Build history of the part. All positions in model axes, mm. Face numbers are marked on the shaded views. Coordinates: 2 decimals unless noted, no trailing zeros. One line per item, written item: value. Start each with the question number.
```python
from build123d import *

# Parameters (mm, degrees)
F0_W     = 135.89
F0_H     = 135.89
F1_DEPTH = 31.75


# Not quite as in the source:
# - a fillet or chamfer that OpenCascade refuses, or shapes differently, is made with other operations: its cross-section is extruded or revolved along the edge and cut away or added


with BuildPart() as f1:
    # F0 (on Top) → F1 (new body)
    with BuildSketch(Plane.XY):
        Rectangle(F0_W, F0_H)
    extrude(amount=F1_DEPTH)

    # F2 (on Front) → F3 (revolve, cut)
    with BuildSketch(Plane.XZ):
        with BuildLine():
            Line((0, 29.21), (0, 31.75))
            Line((0, 31.75), (-44.45, 31.75))
            Line((-44.45, 31.75), (-41.2296488455, 24.8439346628))
            Line((-41.2296488455, 24.8439346628), (-39.4921865174, 29.6175731764))
            ThreePointArc((-39.4921865174, 29.6175731764), (-25.8683470518, 26.5354678002), (-11.9464546442, 25.4))
            Line((-11.9464546442, 25.4), (-11.9464546442, 26.67))
            Line((-11.9464546442, 26.67), (-9.398, 26.67))
            Line((-9.398, 26.67), (-9.398, 29.21))
            Line((-9.398, 29.21), (0, 29.21))
        make_face()
    revolve(axis=Axis((0, 0, 21.6028230067), (0, 0, -1)), mode=Mode.SUBTRACT)

    # F4: fillet of radius 2.54 on 2 edges, made by hand

    # F4_s1 → F4_t2 (revolve, cut)
    with BuildSketch(Plane.XZ):
        with BuildLine():
            ThreePointArc((-9.398, 26.67), (-8.6540512242, 28.4660512242), (-6.858, 29.21))
            Line((-6.858, 29.21), (-9.398, 29.21))
            Line((-9.398, 29.21), (-9.398, 26.67))
        make_face()
    revolve(axis=Axis((0, 0, 29.21), (0, 0, -1)), mode=Mode.SUBTRACT)

    # F4_s3 → F4_t4 (revolve, cut)
    with BuildSketch(Plane.XZ):
        with BuildLine():
            ThreePointArc((-11.9464546442, 25.4), (-11.0167501186, 26.3297045256), (-9.7467501186, 26.67))
            Line((-9.7467501186, 26.67), (-11.9464546442, 26.67))
            Line((-11.9464546442, 26.67), (-11.9464546442, 25.4))
        make_face()
    revolve(axis=Axis((0, 0, 26.67), (0, 0, -1)), mode=Mode.SUBTRACT)


solid = f1.part
```
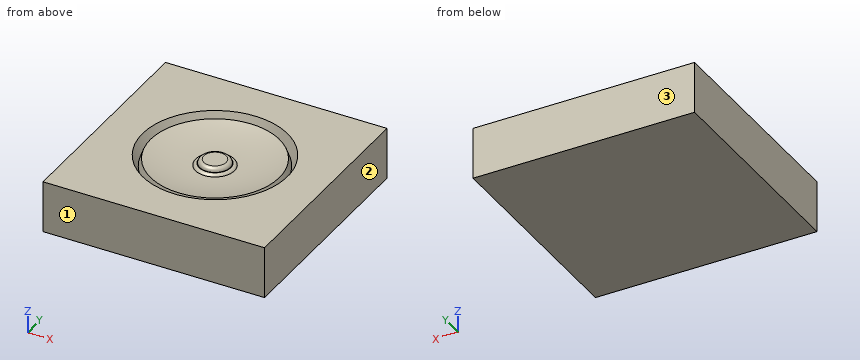
Item 1: Probe probe 1 along Z at (x, y) = (-13, 42); probe 2 along Z at (x, y) = (-28, -18.5). List the from-to ranges inside material, lowest first.
Item 2: Two-plate mould, pull along Y, no slides. Class the marked faces 1, 2 and 3: +Y half, -Y half, draft (parallel to the pull), parting line (faces both ways), or undercut.
Item 3: Drop flat-ended pins along their axis: pin 1 Ø6 at (x, y) = (-3, 3) entering from +Z; pin 2 Ø4 at (x, y) = (-2.5, 16) entering from -Z. Give the stop position or say it passes through.
Worked out:
1. probe 1: z = 0 to 30.71
1. probe 2: z = 0 to 28.03
2. face 1: -Y half
2. face 2: draft
2. face 3: +Y half
3. pin 1: stops at z = 29.21
3. pin 2: stops at z = 0
